from build123d import *

# Parameters (mm, degrees)
F1_DEPTH = 12.7
F2_DEPTH = 5.08
F3_DEPTH = 25.4
F4_R     = 2.54
F5_DEPTH = 3.81


with BuildPart() as f1:
    # F0 (on Top) → F1 (new body)
    with BuildSketch(Plane.XY):
        with BuildLine():
            Line((-12.7, 29.4087881439), (-12.7, 22.4467985298))
            ThreePointArc((-12.7, 22.4467985298), (-6.35, 21.3573107719), (0, 22.4467985298))
            Line((0, 22.4467985298), (0, 29.4087881439))
            ThreePointArc((0, 29.4087881439), (-6.35, 27.7073107719), (-12.7, 29.4087881439))
        make_face()
        with BuildLine():
            ThreePointArc((-25.3555783398, 41.7074999772), (-22.2707409783, 29.9463114553), (-12.7, 22.4467985298))
            Line((-12.7, 22.4467985298), (-12.7, 29.4087881439))
            ThreePointArc((-12.7, 29.4087881439), (-17.5589336819, 34.4365649462), (-19.0203855599, 41.2741035754))
            Line((-19.0203855599, 41.2741035754), (-25.3555783398, 41.7074999772))
        make_face()
        with BuildLine():
            Line((0, 29.4087881439), (0, 22.4467985298))
            ThreePointArc((0, 22.4467985298), (8.8196383991, 28.8840920011), (12.6555783398, 39.1071215667))
            Line((12.6555783398, 39.1071215667), (6.3203855599, 39.5405179684))
            ThreePointArc((6.3203855599, 39.5405179684), (4.4252844056, 33.685462367), (0, 29.4087881439))
        make_face()
    extrude(amount=F1_DEPTH)

    # F0 (on Top) → F2 (join)
    with BuildSketch(Plane.XY):
        with BuildLine():
            Line((-12.7, 22.4467985298), (-12.7, -31.1441666))
            ThreePointArc((-12.7, -31.1441666), (-6.35, -29.4426892281), (0, -31.1441666))
            Line((0, -31.1441666), (0, 22.4467985298))
            ThreePointArc((0, 22.4467985298), (-6.35, 21.3573107719), (-12.7, 22.4467985298))
        make_face()
    extrude(amount=F2_DEPTH)

    # F0 (on Top) → F3 (join)
    with BuildSketch(Plane.XY):
        with BuildLine():
            Line((-12.7, -31.1441666), (-12.7, -42.1426892281))
            Line((-12.7, -42.1426892281), (-6.35, -42.1426892281))
            Line((-6.35, -42.1426892281), (0, -42.1426892281))
            Line((0, -42.1426892281), (0, -31.1441666))
            ThreePointArc((0, -31.1441666), (-6.35, -29.4426892281), (-12.7, -31.1441666))
        make_face()
        with BuildLine():
            Line((-6.35, -42.1426892281), (-12.7, -42.1426892281))
            Line((-12.7, -42.1426892281), (-12.7, -31.1441666))
            ThreePointArc((-12.7, -31.1441666), (-12.7, -53.1412118561), (6.35, -42.1426892281))
            ThreePointArc((6.35, -42.1426892281), (4.6485226281, -35.7926892281), (0, -31.1441666))
            Line((0, -31.1441666), (0, -42.1426892281))
            Line((0, -42.1426892281), (-6.35, -42.1426892281))
        make_face()
    extrude(amount=F3_DEPTH)

    # F4 (on face) → F5 (join)
    with BuildSketch(Plane(origin=(2.7218447995, 39.7866974726, 0), x_dir=(-0.9976681543, 0.0682514019, 0), z_dir=(0.0682514019, 0.9976681543, 0))):
        with Locations((24.9680483851, 6.35)):
            Circle(F4_R)
    extrude(amount=F5_DEPTH)


solid = f1.part
Check sheet for the modelled part. Datum: model origin and axes. Units: mm. A direction names the side the tool comes from. Round coordinates to 2 decimals unless told otherwise and drop trailing zeros. Loops run counter-clockwise (first coordinate to the right, second up) from the corner with the lowest first, then second, coordinate; pieces in that order, holes last.
1. Sectioned sample at D-D on x = 10. Record the boundary of the cut face in (y, z).
2. Gauge pin test, flat ends, axial feed: pin 1 Ø1.5 at (y, z) = (-7, 3) entering from -X; pin 2 Ø2 at (x, y) = (-10, 16) entering from +Z; pin 3 Ø4 at (x, y) = (2.5, -15.5) entering from +Z; pin 4 Ø1 at (x, z) = (3, 8) entering from +Y. Record the tip position at first contact, or that the pin passes through.
3. Sectioned sample at A-A on x = 2.5. Record the boundary of the cut face in (y, z).
4. Mould release check, pull along Y, two halves, no side actions. Record for faces 1 (the flat face through (-7, -6, 0)), 2 (the flat face through (-6, -4, 5.08)), 3 (the flat face through (9.53, 39.32, 6.26)): released by +Y, released by -Y, zero draft, split by the parting line, or undercut.
5. Set-up check for faces 4 (the flat face through (-21.89, 45.29, 6.39)), 5 (the flat face through (-7, 27, 12.7)), 6 (the flat face through (0, -5, 3)), 7 (the flat face through (-12.7, -4, 3)), 8 (the cylindrical face through (-24.477, 43.53, 7.113)): record each of +Z, -Z, +X, -X, +Y, -Y from which the full face is reachable in a straight line by a thin tool's end or side.
6. Sectioned sample at B-B on x = -6.35. Record the boundary of the cut face in (y, z), and give its area (3 significant figures).
7. Scan lines: probe 1 along X at (y, z) = (-15.5, 1.75); probe 2 along Z at (x, y) = (-13, 27.5); probe 3 along X at (y, z) = (40, 9.75). Record each from-to range of solid material in increasing order.
8. Sectioned sample at C-C on y = 3.5. Record the boundary of the cut face in (x, z).
Recorded:
1. outline: (30.63, 0) - (39.29, 0) - (39.29, 12.7) - (30.63, 12.7) - close
2. pin 1: stops at x = -12.7
2. pin 2: stops at z = 5.08
2. pin 3: passes through
2. pin 4: stops at y = 32.39
3. outline: (-51.25, 0) - (-33.03, 0) - (-33.03, 25.4) - (-51.25, 25.4) - close; (23.54, 0) - (31.3, 0) - (31.3, 12.7) - (23.54, 12.7) - close
4. face 1: zero draft
4. face 2: undercut
4. face 3: released by +Y
5. face 4: +Z, -Z, +X, +Y
5. face 5: +Z, +X, -X, +Y
5. face 6: +Z, -Z, +X
5. face 7: +Z, -Z, -X
5. face 8: none
6. outline: (-54.84, 0) - (27.71, 0) - (27.71, 12.7) - (21.36, 12.7) - (21.36, 5.08) - (-29.44, 5.08) - (-29.44, 25.4) - (-54.84, 25.4) - close
6. area: 984 mm2
7. probe 1: x = -12.7 to 0
7. probe 2: z = 0 to 12.7
7. probe 3: x = -25.4 to -19.04
8. outline: (-12.7, 0) - (0, 0) - (0, 5.08) - (-12.7, 5.08) - close
